Geometry check sheet. Reference: the model listing, model coordinates, mm. Face numbers are marked on the shaded views. A direction names the side the tool comes from. Give positions to 0.01 mm unless a question says otherwise; leave off trailing zeros. Write each loop counter-clockwise with the first axis right and the second up, starting at its lowest first coordinate (ties: lowest second). Pieces come first, ordered by that corner, then holes. Notation, with made-up numbers: M 77.25,21.25 L 132.25,21.25 A32 cw 132.25,51.25 Z; hole C 24,62 d8. An arc over 180 degrees is marked long. One line per item, written item: value. Start each with the question number.
1. Cross-section at A-A on y = 0. Record the cut outline in (x, z).
2. Scan lines: line 1 (Y direction, x = -3, z = 0); line 2 (Y direction, x = 8, z = -7.75); line 3 (X direction, y = -6, z = 8.25). Record each from-to range of solid material in increasing order.
3. Release check for a two-part mould opening along Z. For the marked faces 1, 2, 3 and 4 record: pulls with the +Z half, pulls with the -Z half, needs draft (parallel to the pull), parting line crosses it, or undercut.
4. Cross-section at D-D on z = 7. Record the cut outline in (x, y), then the cut area to 3 significant figures.
5. Gauge pin test, flat ends, axial feed: pin 1 (1.3 mm diameter, centred on y = -5, z = 8, fed in from -X); pin 2 (6 mm diameter, centred on x = -6.5, y = 1, fed in from -Z); pin 3 (4 mm diameter, centred on y = 0, z = 0, fed in from +X); pin 4 (2 mm diameter, centred on x = -6, z = -4, fed in from -Y). Record the tip position at first contact, or that the pin passes through.
6. Cross-section at C-C on x = -5.25. Record the cut outline in (y, z), then the cut area to 3 significant figures.
7. Tool access check on the marked faces 5, 6 and 7. Record the directions out of +Z, -Z, +X, -X, +Y, -Y that give a thin tool (end or side, any length) a straight path to the whole face; none if there is none.
from build123d import *
from build123d.topology import SkipClean

# Parameters (mm, degrees)
BASPROSKE_W      = 10
BASPROSKE_H      = 11.25
TOOTHCUT_DEPTH   = 19.791620473
TEETHCUTS_COUNT  = 16
TEETHCUTS_ANGLE  = 337.5
HUBNEAONESKE_R   = 8.4365
HUBNEARONE_DEPTH = 10.0000508
BORSKE_R         = 2.5
BORE_DEPTH       = 20.0000508


with BuildPart() as part:
    # BasProSke → Base-Revolve (revolve)
    with BuildSketch(Plane(origin=(0, 0, 0), x_dir=(1, 0, 0), z_dir=(0, 1, 0)), mode=Mode.PRIVATE) as base_revolve_sk:
        with Locations((5, 5.625)):
            Rectangle(BASPROSKE_W, BASPROSKE_H)
    revolve(base_revolve_sk.sketch.rotate(Axis((-10, 0, 0), (1, 0, 0)), 180), axis=Axis((-10, 0, 0), (1, 0, 0)))

    # TooCutSke → ToothCut (cut, through all)
    with BuildSketch(Plane(origin=(0, 0, 0), x_dir=(0, 0, -1), z_dir=(1, 0, 0))):
        with BuildLine():
            ThreePointArc((0.651061533, 8.411340626), (0, 8.4365), (-0.651061533, 8.411340626))
            ThreePointArc((-0.651061533, 8.411340626), (-1.029874156, 9.883978829), (-1.930926138, 11.108832945))
            ThreePointArc((-1.930926138, 11.108832945), (0, 11.2754), (1.930926138, 11.108832945))
            ThreePointArc((1.930926138, 11.108832945), (1.029874156, 9.883978829), (0.651061533, 8.411340626))
        make_face()
    toothcut = extrude(amount=TOOTHCUT_DEPTH, mode=Mode.SUBTRACT)

    # TeethCuts: ToothCut ×16 about axis
    teethcuts_axis = Axis((-10, 0, 0), (1, 0, 0))
    for i in range(1, TEETHCUTS_COUNT):
        add(toothcut.rotate(teethcuts_axis, i * TEETHCUTS_ANGLE / (TEETHCUTS_COUNT - 1)), mode=Mode.SUBTRACT)

    # HubNeaOneSke → HubNearOne (add)
    with SkipClean():  # the faces are left unmerged after this step: merging them gives an invalid solid
        with BuildSketch(Plane.ZY):
            Circle(HUBNEAONESKE_R)
        extrude(amount=HUBNEARONE_DEPTH)

    # BorSke → Bore (cut, symmetric)
    with SkipClean():  # the faces are left unmerged after this step: merging them gives an invalid solid
        with BuildSketch(Plane(origin=(0, 0, 0), x_dir=(0, 0, -1), z_dir=(1, 0, 0))):
            with Locations(Location((0, 0, 0), (0, 0, 180))):
                Circle(BORSKE_R)
        extrude(amount=BORE_DEPTH, both=True, mode=Mode.SUBTRACT)


solid = part.part
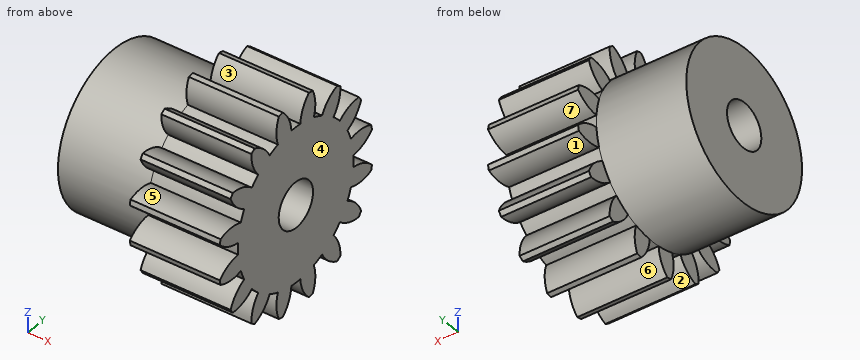
Report:
1. outline: M -10,-8.44 L 10,-8.44 L 10,-2.5 L -10,-2.5 Z; M -10,2.5 L 10,2.5 L 10,8.44 L -10,8.44 Z
2. line 1: y = -8.44 to -2.5, 2.5 to 8.44
2. line 2: y = -6.27 to -3.94, -3.33 to 3.33, 3.94 to 6.27
2. line 3: x = 0 to 10
3. face 1: undercut
3. face 2: pulls with the -Z half
3. face 3: pulls with the +Z half
3. face 4: needs draft
4. outline: M -10,-4.71 L 0,-4.71 L 0,-5.92 L 10,-5.92 L 10,5.92 L 0,5.92 L 0,4.71 L -10,4.71 Z
4. area: 213 mm^2
5. pin 1: stops at x = 0
5. pin 2: stops at z = -8.44
5. pin 3: passes through
5. pin 4: stops at y = -7.89
6. outline: C 0,0 d16.87; hole C 0,0 d5
6. area: 204 mm^2
7. face 5: +X, -X
7. face 6: -Z, +X, -X
7. face 7: +X, -X, +Y
